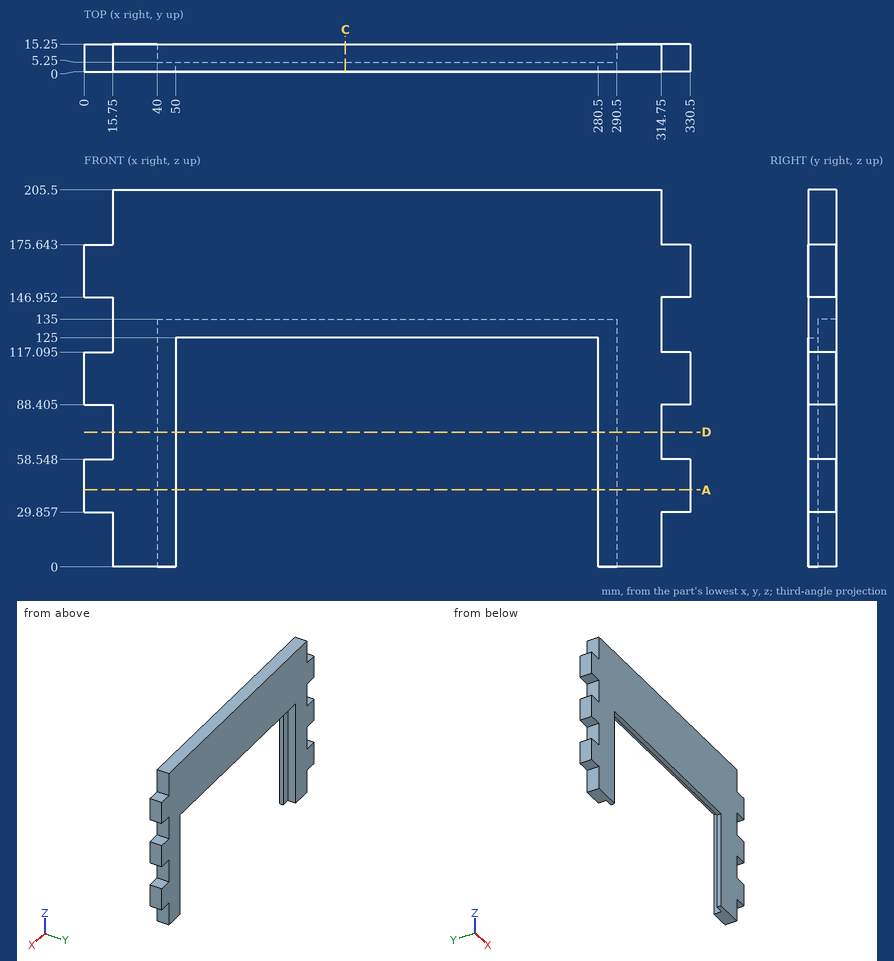
Design review of the part shown in the three views and the two pictorial views. Dimensions are in mm from the part's minimum x, y and z. Give positions to 0.01 mm unless a question says otherwise; leave off trailing zeros. Loops run counter-clockwise (first coordinate to the right, second up) from the corner with the lowest first, then second, coordinate; pieces in that order, holes last. Notation, with made-up numbers: (-39.5, 38) -> (-29.5, 38) arc R19 ccw to (-29.5, 49) -> close; hole circle Ø3 at (-5.5, 14.25). An arc over 180 degrees is marked (long way). Answer as a JSON object with one key per item and string values. Group by question number.
Q1. Take a section at D-D (z = 73.5). Write out the cut boundary in (x, y).
Q2. Insertion check: pin 1 (1 mm diameter, centred on y = 11, z = 176, fed in from -X); pin 2 (4.5 mm diameter, centred on y = 4, z = 68.5, fed in from -X); pin 3 (4.5 mm diameter, centred on y = 6, z = 197.5, fed in from +X); pin 4 (4.5 mm diameter, centred on x = 10, y = 7, fed in from +Z). Each pin has a flat end and moves straight along its axis. Give the tip position at first contact, or say it passes through.
Q3. Wall thickness on line 1 along X through (y, z) = (10.5, 51); line 2 along X through (y, z) = (1.5, 57.5); line 3 along Z through (x, y) = (279.5, 3.5): over which ranges is each line inside the solid? List them lowest first.
Q4. Take a section at A-A (z = 42). Write out the cut boundary in (x, y), plus the area to 4 significant figures.
Q5. Take a section at C-C (x = 142.5). Write out the cut boundary in (y, z).
Answer below:
{
 "1": {"outline": "(15.75, 0) -> (50, 0) -> (50, 5.25) -> (40, 5.25) -> (40, 15.25) -> (15.75, 15.25) -> close; (280.5, 0) -> (314.75, 0) -> (314.75, 15.25) -> (290.5, 15.25) -> (290.5, 5.25) -> (280.5, 5.25) -> close"},
 "2": {"pin 1": "stops at x = 0", "pin 2": "stops at x = 15.75", "pin 3": "stops at x = 314.75", "pin 4": "stops at z = 175.64"},
 "3": {"line 1": "x = 0 to 40, 290.5 to 330.5", "line 2": "x = 0 to 50, 280.5 to 330.5", "line 3": "z = 125 to 205.5"},
 "4": {"outline": "(0, 0) -> (50, 0) -> (50, 5.25) -> (40, 5.25) -> (40, 15.25) -> (0, 15.25) -> close; (280.5, 0) -> (330.5, 0) -> (330.5, 15.25) -> (290.5, 15.25) -> (290.5, 5.25) -> (280.5, 5.25) -> close", "area": "1,325 mm2"},
 "5": {"outline": "(0, 125) -> (5.25, 125) -> (5.25, 135) -> (15.25, 135) -> (15.25, 205.5) -> (0, 205.5) -> close"}
}
